Job drawing, mm, ordinate dimensions from the low corner. One solid piece. A direction names the side the tool comes from. Give positions to 0.01 mm unless a question says otherwise; leave off trailing zeros. Loops run counter-clockwise (first coordinate to the right, second up) from the corner with the lowest first, then second, coordinate; pieces in that order, holes last. Notation, with made-up numbers: M 25,77.25 L 66,77.25 A24 cw 66,103.25 Z; hole C -1,-27.75 d5. An arc over 180 degrees is marked long. Answer as CSV lines item,"result".
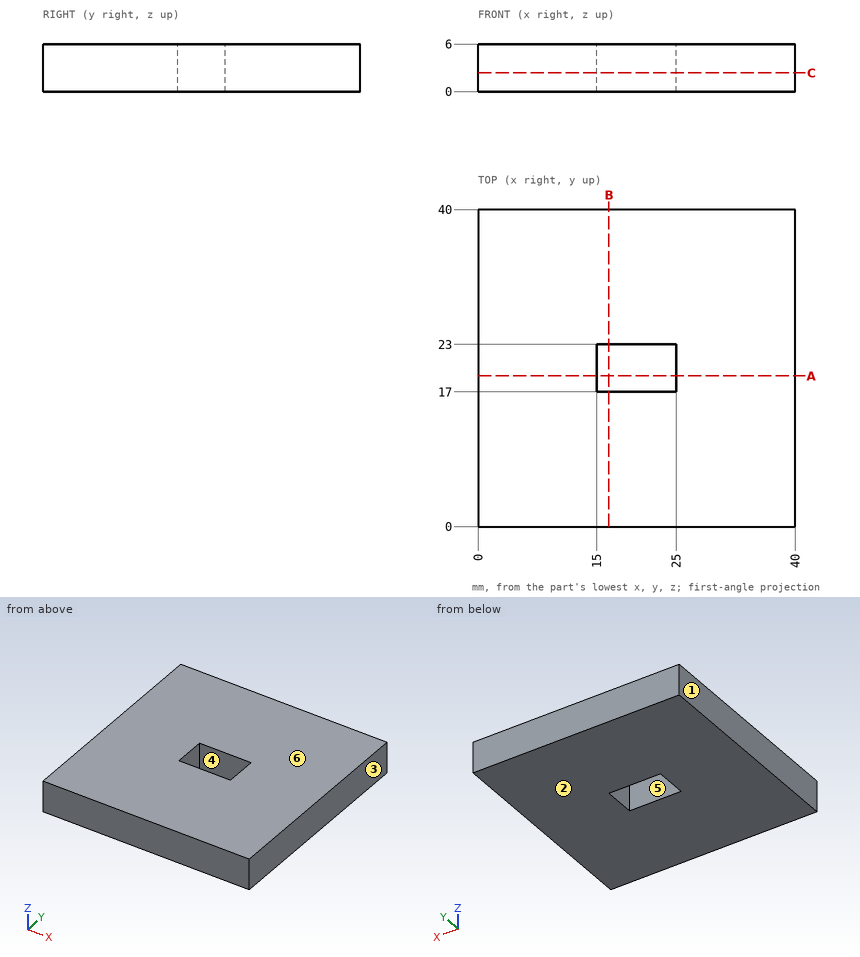
1) Mould opens along X. For the marked faces 1, 2, 3 and 4 say: +X half, -X half, draft (parallel to the pull), parting line (faces both ways), or undercut.
Answer below:
face 1,"-X half"
face 2,"draft"
face 3,"+X half"
face 4,"undercut"
2) Which spindle directions (+Z, -Z, +X, -X, +Y, -Y) get a long thin tool onto all of the face, cutting with end or side? Do the marked faces 5 and 6. Say none if no direction does.
Answer below:
face 5,"+Z, -Z"
face 6,"+Z, +X, -X, +Y, -Y"
3) Band-saw the part on C-C on z = 2.35. Give the cut face in (x, y), and give its area (3 significant figures).
Answer below:
outline,"M 0,0 L 40,0 L 40,40 L 0,40 Z; hole M 15,17 L 25,17 L 25,23 L 15,23 Z"
area,"1,540 mm^2"
4) Band-saw the part on A-A on y = 19. Give the cut face in (x, z).
Answer below:
outline,"M 0,0 L 15,0 L 15,6 L 0,6 Z; M 25,0 L 40,0 L 40,6 L 25,6 Z"
5) Band-saw the part on B-B on x = 16.5. Give the cut face in (y, z).
Answer below:
outline,"M 0,0 L 17,0 L 17,6 L 0,6 Z; M 23,0 L 40,0 L 40,6 L 23,6 Z"
6) Drill centre lines: line 1 (X direction, y = 19, z = 5.1); line 2 (Y direction, x = 17, z = 2.6). Where is each one in solid material? Low to high. Write a range as from..to.
Answer below:
line 1,"x = 0..15, 25..40"
line 2,"y = 0..17, 23..40"
